from build123d import *

# Parameters (mm, degrees)
F0_R     = 4
F0_R_2   = 1.65
F0_R_3   = 2
F1_DEPTH = 6
F2_DEPTH = 5
F3_DEPTH = 3


# Not quite as in the source:
# - a feature names something its author has since deleted; it is built from what else it names


with BuildPart() as f1:
    # F0 (on Top) → F1 (new body)
    with BuildSketch(Plane.XY):
        with BuildLine():
            Line((40, 22.5), (-40, 22.5))
            ThreePointArc((-40, 22.5), (-43.5355339059, 21.0355339059), (-45, 17.5))
            Line((-45, 17.5), (-45, 4))
            Line((-45, 4), (-30, 4))
            Line((-30, 4), (-30, 0))
            Line((-30, 0), (-30, -4))
            Line((-30, -4), (-45, -4))
            Line((-45, -4), (-45, -17.5))
            ThreePointArc((-45, -17.5), (-43.5355339059, -21.0355339059), (-40, -22.5))
            Line((-40, -22.5), (40, -22.5))
            ThreePointArc((40, -22.5), (43.5355339059, -21.0355339059), (45, -17.5))
            Line((45, -17.5), (45, -4))
            Line((45, -4), (30, -4))
            Line((30, -4), (30, 0))
            Line((30, 0), (30, 4))
            Line((30, 4), (45, 4))
            Line((45, 4), (45, 17.5))
            ThreePointArc((45, 17.5), (43.5355339059, 21.0355339059), (40, 22.5))
        make_face()
        with Locations((-17.6776695297, -17.6776695297)):
            Circle(F0_R, mode=Mode.SUBTRACT)
        with Locations((17.6776695297, -17.6776695297)):
            Circle(F0_R, mode=Mode.SUBTRACT)
        with Locations((-17.6776695297, 17.6776695297)):
            Circle(F0_R, mode=Mode.SUBTRACT)
        with Locations((17.6776695297, 17.6776695297)):
            Circle(F0_R, mode=Mode.SUBTRACT)
        Polygon((-30, 4), (-45, 4), (-45, -4), (-30, -4), (-30, 0), align=None)
        with Locations((-37.5, 0)):
            Circle(F0_R_2, mode=Mode.SUBTRACT)
        Polygon((45, -4), (45, 4), (30, 4), (30, 0), (30, -4), align=None)
        with Locations((37.5, 0)):
            Circle(F0_R_2, mode=Mode.SUBTRACT)
        with Locations((-17.6776695297, 17.6776695297)):
            Circle(F0_R)
        with Locations((-17.6776695297, 17.6776695297)):
            Circle(F0_R_2, mode=Mode.SUBTRACT)
        with Locations((-17.6776695297, -17.6776695297)):
            Circle(F0_R)
        with Locations((-17.6776695297, -17.6776695297)):
            Circle(F0_R_3, mode=Mode.SUBTRACT)
        with Locations((17.6776695297, 17.6776695297)):
            Circle(F0_R)
        with Locations((17.6776695297, 17.6776695297)):
            Circle(F0_R_3, mode=Mode.SUBTRACT)
        with Locations((17.6776695297, -17.6776695297)):
            Circle(F0_R)
        with Locations((17.6776695297, -17.6776695297)):
            Circle(F0_R_3, mode=Mode.SUBTRACT)
    extrude(amount=-F1_DEPTH)

    # F0 (on Top) → F2 (cut)
    with BuildSketch(Plane.XY):
        with Locations((-17.6776695297, 17.6776695297)):
            Circle(F0_R)
        with Locations((-17.6776695297, 17.6776695297)):
            Circle(F0_R_2, mode=Mode.SUBTRACT)
        with Locations((-17.6776695297, 17.6776695297)):
            Circle(F0_R_2)
        with Locations((-17.6776695297, -17.6776695297)):
            Circle(F0_R)
        with Locations((-17.6776695297, -17.6776695297)):
            Circle(F0_R_3, mode=Mode.SUBTRACT)
        with Locations((17.6776695297, -17.6776695297)):
            Circle(F0_R)
        with Locations((17.6776695297, -17.6776695297)):
            Circle(F0_R_3, mode=Mode.SUBTRACT)
        with Locations((17.6776695297, 17.6776695297)):
            Circle(F0_R)
        with Locations((17.6776695297, 17.6776695297)):
            Circle(F0_R_3, mode=Mode.SUBTRACT)
    extrude(amount=-F2_DEPTH, mode=Mode.SUBTRACT)

    # F0 (on Top) → F3 (join)
    with BuildSketch(Plane.XY):
        Polygon((-30, 4), (-45, 4), (-45, -4), (-30, -4), (-30, 0), align=None)
        with Locations((-37.5, 0)):
            Circle(F0_R_2, mode=Mode.SUBTRACT)
        Polygon((45, -4), (45, 4), (30, 4), (30, 0), (30, -4), align=None)
        with Locations((37.5, 0)):
            Circle(F0_R_2, mode=Mode.SUBTRACT)
    extrude(amount=F3_DEPTH)


solid = f1.part
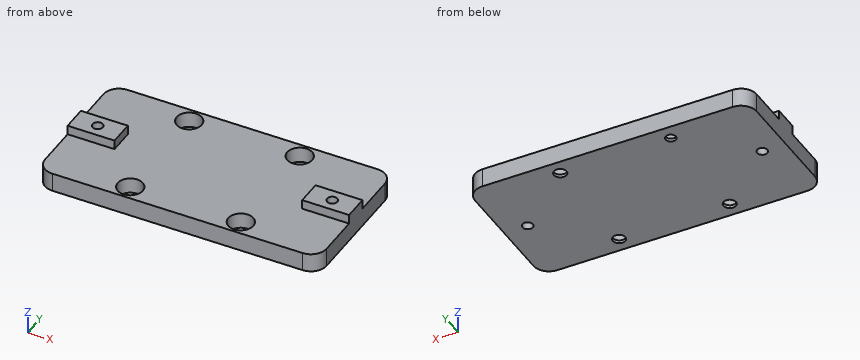
Verification items for the finished model (mm, model axes). Give positions to 0.01 mm unless a question says otherwise; leave off trailing zeros. Write each loop counter-clockwise with the first axis right and the second up, starting at its lowest first coordinate (ties: lowest second). Pieces come first, ordered by that corner, then holes.
(1) Cross-section at B-B (y = 0). Enter the section's corners in (x, z).
(2) Cross-section at D-D (z = -4). Enter the section's corners in (x, y).
(3) Material ranges on line 1 (Y direction, x = 37.5, z = 0.85); line 2 (Y direction, x = 37.5, z = -4.7); line 3 (Y direction, x = 17, z = -2.5), recorded low to high.
(4) Gauge pin test, flat ends, axial feed: pin 1 (1.5 mm diameter, centred on x = 8, y = -14.5, fed in from +Z); pin 2 (3 mm diameter, centred on x = 37.5, y = 0, fed in from +Z); pin 3 (1.5 mm diameter, centred on x = 40.5, z = 2, fed in from -Y); pin 4 (1.5 mm diameter, centred on x = 40, z = 1, fed in from +Y). Record the tip position at first contact, or that the pin passes through.
(5) Cross-section at A-A (x = 37.5). Enter the section's corners in (y, z), plus the area to 3 significant figures.
(6) Cross-section at C-C (x = -31.5). Enter the section's corners in (y, z), plus the area to 3 significant figures.
Worked out:
1. outline: (-45, -6) - (-39.15, -6) - (-39.15, 3) - (-45, 3) - close; (-35.85, -6) - (35.85, -6) - (35.85, 3) - (30, 3) - (30, 0) - (-30, 0) - (-30, 3) - (-35.85, 3) - close; (39.15, -6) - (45, -6) - (45, 3) - (39.15, 3) - close
2. outline: (-45, -17.5) arc R5 ccw to (-40, -22.5) - (40, -22.5) arc R5 ccw to (45, -17.5) - (45, 17.5) arc R5 ccw to (40, 22.5) - (-40, 22.5) arc R5 ccw to (-45, 17.5) - close; hole circle Ø3.3 at (-37.5, 0); hole circle Ø8 at (-17.68, -17.68); hole circle Ø8 at (-17.68, 17.68); hole circle Ø8 at (17.68, -17.68); hole circle Ø8 at (17.68, 17.68); hole circle Ø3.3 at (37.5, 0)
3. line 1: y = -4 to -1.65, 1.65 to 4
3. line 2: y = -22.5 to -1.65, 1.65 to 22.5
3. line 3: y = -22.5 to -21.62, -13.74 to 13.74, 21.62 to 22.5
4. pin 1: stops at z = 0
4. pin 2: passes through
4. pin 3: stops at y = -4
4. pin 4: stops at y = 4
5. outline: (-22.5, -6) - (-1.65, -6) - (-1.65, 3) - (-4, 3) - (-4, 0) - (-22.5, 0) - close; (1.65, -6) - (22.5, -6) - (22.5, 0) - (4, 0) - (4, 3) - (1.65, 3) - close
5. area: 264 mm2
6. outline: (-22.5, -6) - (22.5, -6) - (22.5, 0) - (4, 0) - (4, 3) - (-4, 3) - (-4, 0) - (-22.5, 0) - close
6. area: 294 mm2
